The model under review builds one solid part; all positions refer to its coordinate system, in mm. A direction names the side the tool comes from. Coordinates: 2 decimals unless noted, no trailing zeros. Order: outer loops, then holes, each group sorted by start corner. A loop starts at its lowest first (then second) coordinate and runs counter-clockwise, first axis right, second up. Notation, with made-up numbers: (71.5, 57) -> (99.5, 57) arc R32 ccw to (99.5, 87) -> close; hole circle Ø8 at (35.5, -25). An arc over 180 degrees is marked (long way). Use one line per item in the form item = value.
Autodesk Inventor part; units mm, degrees
ref_plane "YZ Plane" through (0, 0, 0) normal (1, 0, 0) x (0, 1, 0)
ref_plane "XZ Plane" through (0, 0, 0) normal (0, 1, 0) x (-1, 0, 0)
ref_plane "XY Plane" through (0, 0, 0) normal (0, 0, 1) x (1, 0, 0)
sketch "Skizze6" plane through (0, 0, 0) normal (1, 0, 0) x (0, 1, 0)
  line L0 (-253.2103, 0) -> (-253.2103, 5)
  line L1 (-253.2103, 5) -> (-168.2103, 5)
  line L2 (-168.2103, 5) -> (-168.2103, 1.6557)
  line L3 (-168.2103, 1.6557) -> (-166.2103, 1.6557)
  line L4 (-166.2103, 1.6557) -> (-164.9254, 2)
  line L5 (-164.9254, 2) -> (-163.2103, 2)
  line L6 (-163.2103, 2) -> (-163.2103, 0)
  line L7 (-163.2103, 0) -> (-253.2103, 0)
  point P0 (0, 0)
  dimension "d31" = 5
  dimension "d32" = 85
  dimension "d33" = 5
  dimension "d34" = 2
  dimension "d35" = 15
  dimension "d36" = 2
revolve "Umdrehung1" add sketch "Skizze6" angle 360 about axis through (0, -163.2103, 0) along (0, -1, 0)
thread "Gewinde2"
fillet "Rundung6" radius 0.4 2 edges at (0, -166.2103, -1.6557) (0, -168.2103, -1.6557)
properties part number "TS_V1_Fallmagazin_Blech_int"
Item 1: Tool access review of faces 1 (the face through (-4.88, -210.12, -1.08)), 2 (the face through (-1.01, -167.03, -1.31)): name each direction out of +Z, -Z, +X, -X, +Y, -Y from which nothing blocks a thin tool from reaching the whole face with its end or side.
Results found:
face_1 = +Y, -Y
face_2 = none
Item 2: Draft analysis for pull direction Y (two halves, no side actions). For faces 3 (the face through (-1.05, -165.95, -1.37)), 4 (the face through (-2, -164, 0)), 5 (the face through (1, -168.21, 2)), state which applies: released by +Y, released by -Y, zero draft, split by the parting line, or undercut.
Results found:
face_3 = undercut
face_4 = zero draft
face_5 = released by +Y
Item 3: We need section B-B (z = 3.5). Write out the cut boundary in (x, y).
Results found:
outline = (-3.57, -253.21) -> (3.57, -253.21) -> (3.57, -168.21) -> (-3.57, -168.21) -> close
Item 4: Clearance check with flat-ended pins moving along their axes: pin 1 (3 mm diameter, centred on x = -2.5, z = 2.5, fed in from +Y); pin 2 (4 mm diameter, centred on x = 4, y = -184.5, fed in from +Z); pin 3 (6 mm diameter, centred on x = -3.5, y = -229, fed in from +Z). State where each tip first meets the part, or that it passes through.
Results found:
pin_1 = -168.21
pin_2 = 4.58
pin_3 = 4.97
Item 5: To check wall thickness, follow L1, parallel to Y at x = 0.25, z = -4; L2, parallel to Z at x = -0.25, y = -241.5; L3, parallel to X at y = -185, z = -1.25. State the ranges of each line that lie inside material, in increasing order. Write a range as from..to.
Results found:
L1 = -253.21..-168.21
L2 = -4.99..4.99
L3 = -4.84..4.84
Item 6: We need section A-A (y = -217). Write out the cut boundary in (x, z).
Results found:
outline = circle Ø10 at (0, 0)
